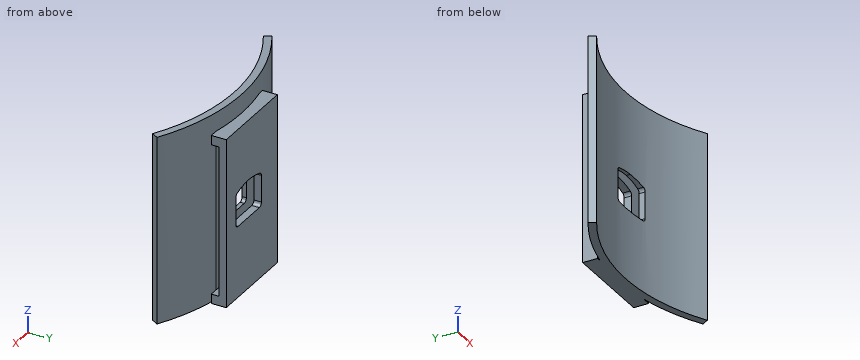
```python
from build123d import *

# Parameters (mm, degrees)
BOX002_W                    = 23
BOX002_H                    = 2
BOX002_DEPTH                = 40
EXTRUDE_DEPTH               = 6
EXTRUDE001_DEPTH            = 6
THICKNESS_T                 = 1
BOX001_W                    = 24
BOX001_H                    = 4
BOX001_DEPTH                = 45
CYLINDER001_W               = 52
CYLINDER001_H               = 50
CYLINDER001_ANGLE           = 60
CYLINDER001_PLACEMENT_ANGLE = 60
CYLINDER_W                  = 54
CYLINDER_H                  = 50
CYLINDER_ANGLE              = 60
CYLINDER_PLACEMENT_ANGLE    = 60


with BuildPart() as slot:
    # Box002 → Box002 (new body)
    with BuildSketch(Plane(origin=(-1, 44, 2.5), x_dir=(1, 0, 0), z_dir=(0, 0, 1))):
        with Locations((11.5, 1)):
            Rectangle(BOX002_W, BOX002_H)
    extrude(amount=BOX002_DEPTH)


with BuildPart() as extrude_body:
    with BuildSketch(Plane(origin=(8.5, 45, 6), x_dir=(1, 0, 0), z_dir=(0, 1, 0))):
        with BuildLine():
            Line((5, 4), (-5, 4))
            Line((-5, 4), (-5, -3.142136))
            ThreePointArc((-5, -3.142136), (-2.53653, -3.783978), (0, -4))
            ThreePointArc((0, -4), (2.53653, -3.783978), (5, -3.142136))
            Line((5, -3.142136), (5, 4))
        make_face()
    extrude(amount=EXTRUDE_DEPTH)


with BuildPart() as extrude001:
    with BuildSketch(Plane(origin=(8.5, 45, 6), x_dir=(1, 0, 0), z_dir=(0, 1, 0))):
        with BuildLine():
            Line((5, 4), (-5, 4))
            Line((-5, 4), (-5, -3.142136))
            ThreePointArc((-5, -3.142136), (-2.53653, -3.783978), (0, -4))
            ThreePointArc((0, -4), (2.53653, -3.783978), (5, -3.142136))
            Line((5, -3.142136), (5, 4))
        make_face()
    extrude(amount=EXTRUDE001_DEPTH)


with BuildPart() as pin_opening:
    # Thickness base: copy of Extrude body
    add(extrude_body.part)

    # Thickness
    thickness_openings = [pin_opening.faces().sort_by_distance(p)[0] for p in [
        (8.5, 51, 5.862901),
    ]]
    offset(amount=THICKNESS_T, openings=thickness_openings)

    # Fusion002: union Extrude body, Extrude001
    add(extrude_body.part)
    add(extrude001.part)


with BuildPart() as pin_opening_1:
    # Fusion002 placement: moved
    add(pin_opening.part.moved(Location((2, -3, 18))))


with BuildPart() as latch:
    # Box001 → Box001 (new body)
    with BuildSketch(Plane(origin=(-3, 44, 0), x_dir=(1, 0, 0), z_dir=(0, 0, 1))):
        with Locations((12, 2)):
            Rectangle(BOX001_W, BOX001_H)
    extrude(amount=BOX001_DEPTH)


with BuildPart() as bottle_wall001:
    # Cylinder001 → Cylinder001 (revolve)
    with BuildSketch(Plane.XZ):
        with Locations((26, 25)):
            Rectangle(CYLINDER001_W, CYLINDER001_H)
    revolve(axis=Axis((0, 0, 0), (0, 0, 1)), revolution_arc=CYLINDER001_ANGLE)


with BuildPart() as bottle_wall001_1:
    # Cylinder001 placement: moved
    add(bottle_wall001.part.moved(Location((8.5, -7, 0))).rotate(Axis((8.5, -7, 0), (0, 0, 1)), CYLINDER001_PLACEMENT_ANGLE))


with BuildPart() as cut004:
    # Cylinder → Cylinder (revolve)
    with BuildSketch(Plane.XZ):
        with Locations((27, 25)):
            Rectangle(CYLINDER_W, CYLINDER_H)
    revolve(axis=Axis((0, 0, 0), (0, 0, 1)), revolution_arc=CYLINDER_ANGLE)


with BuildPart() as cut004_1:
    # Cylinder placement: moved
    add(cut004.part.moved(Location((8.5, -7, 0))).rotate(Axis((8.5, -7, 0), (0, 0, 1)), CYLINDER_PLACEMENT_ANGLE))

    # Cut: cut bottle_wall001
    add(bottle_wall001_1.part, mode=Mode.SUBTRACT)


with BuildPart() as cut004_2:
    # Cut placement: moved
    add(cut004_1.part.moved(Location((0, -2, 0))))

    # Fusion: union latch
    add(latch.part)

    # Fusion001: union latch
    add(latch.part)

    # Cut003: cut pin opening
    add(pin_opening_1.part, mode=Mode.SUBTRACT)

    # Cut004: cut slot
    add(slot.part, mode=Mode.SUBTRACT)


solid = cut004_2.part
```
Geometry check sheet. Reference: the model listing, model coordinates, mm. Coordinates: 2 decimals unless noted, no trailing zeros. Order: outer loops, then holes, each group sorted by start corner. A loop starts at its lowest first (then second) coordinate and runs counter-clockwise, first axis right, second up.
Q1. Depth check by flat-ended pin: pin 1 Ø11 at (x, z) = (14, 21.5) entering from -Y; pin 2 Ø2 at (x, y) = (15, 46.5) entering from +Z; pin 3 Ø1.6 at (y, z) = (47, 23.5) entering from -X. Enter the tip coordinate at first touch or a pass-through.
Reply:
pin 1: stops at y = 41.82
pin 2: stops at z = 45
pin 3: stops at x = -3
Q2. Sectioned sample at D-D on z = 15. Record the cut outline in (x, y), and give its area (3 significant figures).
Reply:
outline: (-18.5, 37.77) - (-17.5, 36.03) arc R52 cw to (34.5, 36.03) - (35.5, 37.77) arc R54 ccw to (18.84, 44) - (-1, 44) - (-1, 46) - (21, 46) - (21, 48) - (-3, 48) - (-3, 44) - (-1.84, 44) arc R54 ccw to start
area: 149 mm2
Q3. Sectioned sample at A-A on y = 40.25. Record the cut outline in (x, z), and give its area (3 significant figures).
Reply:
outline: (-13.65, 0) - (-8.19, 0) - (-8.19, 50) - (-13.65, 50) - close; (25.19, 0) - (30.65, 0) - (30.65, 50) - (25.19, 50) - close
area: 546 mm2
Q4. Sectioned sample at B-B on x = 9.5. Record the cut outline in (y, z), and give its area (3 significant figures).
Reply:
outline: (42.99, 0) - (48, 0) - (48, 19) - (46, 19) - (46, 2.5) - (44, 2.5) - (44, 19) - (42.99, 19) - close; (42.99, 28.97) - (44, 28.97) - (44, 42.5) - (46, 42.5) - (46, 28.97) - (48, 28.97) - (48, 45) - (44.99, 45) - (44.99, 50) - (42.99, 50) - close
area: 125 mm2
Q5. Sectioned sample at C-C on y = 47. Record the cut outline in (x, z).
Reply:
outline: (-3, 0) - (21, 0) - (21, 45) - (-3, 45) - close; hole (4.5, 20) arc R1 ccw to (5.5, 19) - (15.5, 19) arc R1 ccw to (16.5, 20) - (16.5, 27.14) arc R1 ccw to (15.83, 28.08) arc R16 ccw to (10.5, 29) arc R16 ccw to (5.17, 28.08) arc R1 ccw to (4.5, 27.14) - close
Q6. Thickness scan on probe 1 along Y at (x, z) = (8, 16.5); probe 2 along Z at (x, y) = (1, 47.75); probe 3 along Y at (x, z) = (16.5, 34.5). Record the ranges inside material, lowest first.
Reply:
probe 1: y = 43 to 44, 46 to 48
probe 2: z = 0 to 45
probe 3: y = 42.38 to 44, 46 to 48
